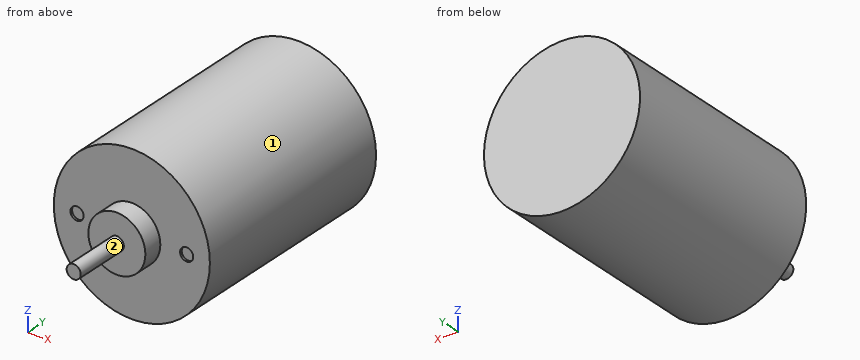
```python
from build123d import *

# Parameters (mm, degrees)
F0_R     = 17.8
F1_DEPTH = 50
F2_R     = 6.5
F3_DEPTH = 4.5
F4_R     = 1.6
F5_DEPTH = 13
F6_R     = 1.5
F7_DEPTH = 0.5


with BuildPart() as f1:
    # F0 (on Front) → F1 (new body)
    with BuildSketch(Plane.XZ):
        Circle(F0_R)
    extrude(amount=F1_DEPTH)

    # F2 (on face) → F3 (join)
    with BuildSketch(Plane.XZ.offset(50)):
        Circle(F2_R)
    extrude(amount=F3_DEPTH)

    # F4 (on face) → F5 (join)
    with BuildSketch(Plane.XZ.offset(54.5)):
        Circle(F4_R)
    extrude(amount=F5_DEPTH)

    # F6 (on face) → F7 (cut)
    with BuildSketch(Plane.XZ.offset(50)):
        with Locations((-12.5, 0)):
            Circle(F6_R)
        with Locations((12.5, 0)):
            Circle(F6_R)
    extrude(amount=-F7_DEPTH, mode=Mode.SUBTRACT)


solid = f1.part
```
Work out the finished part from the listing and answer in its coordinate system (mm). Face numbers are marked on the shaded views. A direction names the side the tool comes from. Round coordinates to 2 decimals unless told otherwise and drop trailing zeros. Loops run counter-clockwise (first coordinate to the right, second up) from the corner with the lowest first, then second, coordinate; pieces in that order, holes last. Notation, with made-up numbers: M 55.25,-15.5 L 85.25,-15.5 A18 cw 85.25,-9.5 Z; hole C 8,61 d10. An arc over 180 degrees is marked long. Use CSV: the item, a comma, the result in double quotes.
Q1. Section A-A, the plane x = 0 is taken. Determine the outline of the cut face in (y, z).
Determined:
outline,"M -67.5,-1.6 L -54.5,-1.6 L -54.5,-6.5 L -50,-6.5 L -50,-17.8 L 0,-17.8 L 0,17.8 L -50,17.8 L -50,6.5 L -54.5,6.5 L -54.5,1.6 L -67.5,1.6 Z"
Q2. Section C-C, the plane y = -63 is taken. Determine the outline of the cut face in (x, z), then the cut area to 3 significant figures.
Determined:
outline,"C 0,0 d3.2"
area,"8.04 mm2"
Q3. Each of these flat-tipped pins is pushed along its axis until it touches: pin 1 (6 mm diameter, centred on x = -5.5, y = -8, fed in from -Z); pin 2 (10 mm diameter, centred on y = -31.5, z = -8.5, fed in from -X); pin 3 (8 mm diameter, centred on x = -14, y = -48, fed in from +Z). Where does it stop, or does it pass through?
Determined:
pin 1,"z = -17.62"
pin 2,"x = -17.45"
pin 3,"z = 14.73"
Q4. Consider L1, parallel to Y at x = 2, z = -14; L2, parallel to Z at x = -12.5, y = -49.55; L3, parallel to Y at x = -5.5, z = -2. Determine where each line is inside the solid, lowest interval first.
Determined:
L1,"-50 to 0"
L2,"-12.67 to -1.5, 1.5 to 12.67"
L3,"-54.5 to 0"
Q5. Section B-B, the plane z = 0 is taken. Determine the outline of the cut face in (x, y), then the cut area to 3 significant figures.
Determined:
outline,"M -17.8,-50 L -14,-50 L -14,-49.5 L -11,-49.5 L -11,-50 L -6.5,-50 L -6.5,-54.5 L -1.6,-54.5 L -1.6,-67.5 L 1.6,-67.5 L 1.6,-54.5 L 6.5,-54.5 L 6.5,-50 L 11,-50 L 11,-49.5 L 14,-49.5 L 14,-50 L 17.8,-50 L 17.8,0 L -17.8,0 Z"
area,"1,880 mm2"
Q6. A tool of negligible diameter and unlimited length cuts with its end or side. For the marked faces 1 and 2, from which of +Z, -Z, +X, -X, +Y, -Y can it reach the whole face along a straight path? Write none if from no direction.
Determined:
face 1,"+Y, -Y"
face 2,"-Y"
Q7. Section D-D, the plane x = 12.5 is taken. Determine the outline of the cut face in (y, z).
Determined:
outline,"M -50,-12.67 L 0,-12.67 L 0,12.67 L -50,12.67 L -50,1.5 L -49.5,1.5 L -49.5,-1.5 L -50,-1.5 Z"
